from build123d import *

# Parameters (mm, degrees)
BOSS_EXTRUDE1_DEPTH = 3
SKETCH2_R           = 3.0000000000000013
BOSS_EXTRUDE2_DEPTH = 65
SKETCH14_R          = 2.999999999999994
CUT_EXTRUDE1_DEPTH  = 8
SKETCH15_R          = 2.999999999999994
CUT_EXTRUDE2_DEPTH  = 10
SKETCH16_R          = 2.999999999999994
CUT_EXTRUDE3_DEPTH  = 10
SKETCH17_R          = 3.0000000000000013
CUT_EXTRUDE4_DEPTH  = 7
CUT_EXTRUDE5_DEPTH  = 7
SKETCH19_R          = 3.0000000000000013
BOSS_EXTRUDE3_DEPTH = 65
SKETCH13_R          = 1.500000000000004
CUT_EXTRUDE7_DEPTH  = 77.29711659034044
SKETCH20_R          = 1.5000000000000042
CUT_EXTRUDE8_DEPTH  = 77.29711659034045
FILLET1_R           = 1
SKETCH21_R          = 1.5000000000000075
BOSS_EXTRUDE4_DEPTH = 65
SKETCH22_W          = 5.918541019528025
SKETCH22_H          = 2.806652575268912
CUT_EXTRUDE9_DEPTH  = 77.29711659034044


with BuildPart() as part:
    # Sketch1 → Boss-Extrude1 (new body)
    with BuildSketch(Plane(origin=(0, 0, 0), x_dir=(1, 0, 0), z_dir=(0, 1, 0))):
        Polygon((-32.50000000000001, 36.49999999999999), (32.49999999999999, 36.49999999999999), (32.500000000000014, -36.50000000000001), (-32.5, -36.50000000000001), align=None)
    extrude(amount=BOSS_EXTRUDE1_DEPTH)

    # Sketch2 → Boss-Extrude2 (add, through all)
    with BuildSketch(Plane(origin=(32.5, 0, -9.27e-15), x_dir=(0, 0, -1), z_dir=(1, 0, 0))):
        with Locations((-36.500000000000014, 0)):
            Circle(SKETCH2_R)
    extrude(amount=-BOSS_EXTRUDE2_DEPTH)

    # Sketch14 → Cut-Extrude1 (cut)
    with BuildSketch(Plane.ZY.offset(24.500000000000004)):
        with Locations((36.500000000000014, 0)):
            Circle(SKETCH14_R)
    extrude(amount=CUT_EXTRUDE1_DEPTH, mode=Mode.SUBTRACT)

    # Sketch15 → Cut-Extrude2 (cut)
    with BuildSketch(Plane.ZY.offset(4.5000000000000036)):
        with Locations((36.500000000000014, 0)):
            Circle(SKETCH15_R)
    extrude(amount=CUT_EXTRUDE2_DEPTH, mode=Mode.SUBTRACT)

    # Sketch16 → Cut-Extrude3 (cut)
    with BuildSketch(Plane.ZY.offset(-15.499999999999996)):
        with Locations((36.500000000000014, 0)):
            Circle(SKETCH16_R)
    extrude(amount=CUT_EXTRUDE3_DEPTH, mode=Mode.SUBTRACT)

    # Sketch17 → Cut-Extrude4 (cut)
    with BuildSketch(Plane(origin=(32.5, 0, -9.27e-15), x_dir=(-1.9e-16, 0, -1), z_dir=(1, 0, -1.9e-16))):
        with Locations((-36.500000000000014, 0)):
            Circle(SKETCH17_R)
    extrude(amount=-CUT_EXTRUDE4_DEPTH, mode=Mode.SUBTRACT)

    # Sketch18 → Cut-Extrude5 (cut)
    with BuildSketch(Plane(origin=(0, 3, 0), x_dir=(1, 0, 0), z_dir=(0, 1, 0))):
        with BuildLine():
            Line((-30.50000000000002, 10.499999999999995), (-30.50000000000002, 9.500000000000002))
            ThreePointArc((-30.50000000000002, 9.500000000000002), (-28.500000000000018, 7.499999999999998), (-26.500000000000018, 9.500000000000002))
            Line((-26.500000000000018, 9.500000000000002), (-26.500000000000018, 10.499999999999995))
            ThreePointArc((-26.500000000000018, 10.499999999999995), (-28.500000000000018, 12.499999999999995), (-30.50000000000002, 10.499999999999995))
        make_face()
        with BuildLine():
            Line((26.5, -29.500000000000007), (26.5, -30.5))
            ThreePointArc((26.5, -30.5), (28.499999999999993, -32.49999999999999), (30.49999999999999, -30.5))
            Line((30.49999999999999, -30.5), (30.49999999999999, -29.500000000000007))
            ThreePointArc((30.49999999999999, -29.500000000000007), (28.499999999999993, -27.50000000000001), (26.5, -29.500000000000007))
        make_face()
    extrude(amount=-CUT_EXTRUDE5_DEPTH, mode=Mode.SUBTRACT)

    # Sketch19 → Boss-Extrude3 (add)
    with BuildSketch(Plane.ZY.offset(32.50000000000001)):
        with Locations((-28.500000000000004, 2.999999999999999)):
            Circle(SKETCH19_R)
    extrude(amount=-BOSS_EXTRUDE3_DEPTH)

    # Sketch13 → Cut-Extrude7 (cut, through all)
    with BuildSketch(Plane(origin=(32.5, 0, -9.27e-15), x_dir=(0, 0, -1), z_dir=(1, 0, 0))):
        with Locations((-36.500000000000014, 0)):
            Circle(SKETCH13_R)
    extrude(amount=-CUT_EXTRUDE7_DEPTH, mode=Mode.SUBTRACT)

    # Sketch20 → Cut-Extrude8 (cut, through all)
    with BuildSketch(Plane.ZY.offset(32.50000000000001)):
        with Locations((-28.5, 2.999999999999999)):
            Circle(SKETCH20_R)
    extrude(amount=-CUT_EXTRUDE8_DEPTH, mode=Mode.SUBTRACT)

    # Fillet1
    fillet1_edges = [part.edges().sort_by_distance(p)[0] for p in [
        (-28.5, 3, 36.50000000000001),
        (-9.5, 3, 36.50000000000001),
        (10.500000000000004, 3, 36.50000000000001),
        (29.00000000000001, 3, 36.50000000000001),
    ]]
    fillet(fillet1_edges, radius=FILLET1_R)

    # Sketch21 → Boss-Extrude4 (add, through all)
    with BuildSketch(Plane.ZY.offset(32.50000000000001)):
        with BuildLine():
            Line((-33.50000000000001, 0), (-23.500000000000007, 0))
            Line((-23.500000000000007, 0), (-23.500000000000007, 3.9999999999999933))
            ThreePointArc((-23.500000000000007, 3.9999999999999933), (-23.79289321881346, 4.707106781186548), (-24.500000000000014, 5))
            Line((-24.500000000000014, 5), (-32.5, 5))
            ThreePointArc((-32.5, 5), (-33.20710678118655, 4.707106781186548), (-33.50000000000001, 3.9999999999999933))
            Line((-33.50000000000001, 3.9999999999999933), (-33.50000000000001, 0))
        make_face()
        with Locations((-28.500000000000004, 2.999999999999999)):
            Circle(SKETCH21_R, mode=Mode.SUBTRACT)
    extrude(amount=-BOSS_EXTRUDE4_DEPTH)

    # Sketch22 → Cut-Extrude9 (cut, through all)
    with BuildSketch(Plane(origin=(32.5, 0, -9.27e-15), x_dir=(-2.9e-16, 0, -1), z_dir=(1, 0, -2.9e-16))):
        with Locations((28.341236521014125, 6.4033262876344565)):
            Rectangle(SKETCH22_W, SKETCH22_H)
    extrude(amount=-CUT_EXTRUDE9_DEPTH, mode=Mode.SUBTRACT)


solid = part.part
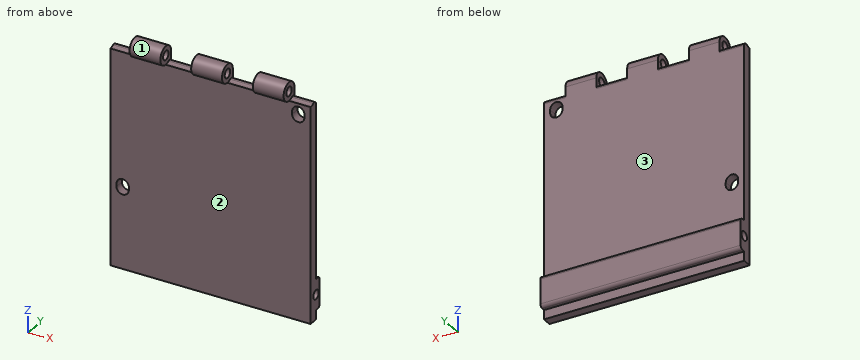
Here's how the part is built. I have some questions about the finished solid (model axes, mm). Face numbers are marked on the shaded views. A direction names the side the tool comes from. Coordinates: 2 decimals unless noted, no trailing zeros. Loops run counter-clockwise (first coordinate to the right, second up) from the corner with the lowest first, then second, coordinate; pieces in that order, holes last.
1. I need wall thicknesses on L1, parallel to Y at x = -19, z = 36.5; L2, parallel to Y at x = -13, z = -28.5; L3, parallel to Y at x = -5, z = 7.5. Which ranges of each line are inside material? Lowest first, please.
2. For P1, Ø0.5, axis at x = -3, y = 3.5, coming from the -Z side; P2, Ø2, axis at x = -2.5, z = -17, coming from the +Y side; P3, Ø6, axis at x = 12.5, z = 14.5, coming from the -Y side, each with a flat end and sliding along its axis, tell me the tip position at first contact or that it passes through.
3. Imagine slicing it at B-B, the plane x = 12. Please give me the cut outline in (y, z).
4. Imagine slicing it at A-A, the plane x = -28.5. Please give me the cut outline in (y, z), and give its area (3 significant figures).
5. Imagine slicing it at C-C, the plane z = 18. Please give me the cut outline in (x, y).
6. For the marked faces 1, 2 and 3, which set-ups out of +Z, -Z, +X, -X, +Y, -Y let a thin tool reach every point of the face, with its end or its side?
Taken from the geometry:
1. L1: y = -3 to -1.5, 1.5 to 3
1. L2: y = 0 to 1.5, 4.5 to 5
1. L3: y = 0 to 3
2. P1: stops at z = -33.5
2. P2: stops at y = 3
2. P3: stops at y = 0
3. outline: (0, -36.5) - (3, -36.5) - (3, -33.5) - (4, -33.5) arc R1 ccw to (5, -32.5) - (5, -24.5) arc R1 ccw to (4, -23.5) - (3, -23.5) - (3, 33.04) arc R1 ccw to (1.5, 33.9) arc R3 cw to (0, 33.5) - close; hole circle Ø3 at (3, -28.5)
4. outline: (0, -36.5) - (3, -36.5) - (3, -33.5) - (4, -33.5) arc R1 ccw to (5, -32.5) - (5, -24.5) arc R1 ccw to (4, -23.5) - (3, -23.5) - (3, -12.5) - (0, -12.5) - close; (0, -7.5) - (3, -7.5) - (3, 33.04) arc R1 ccw to (1.5, 33.9) arc R3 cw to (0, 33.5) - close; hole circle Ø3 at (3, -28.5)
4. area: 208 mm2
5. outline: (-32.5, 0) - (32.5, 0) - (32.5, 3) - (-32.5, 3) - close
6. face 1: +X, -X
6. face 2: -Z, +X, -X, -Y
6. face 3: +Z, +X, -X, +Y
